Design review of the part shown in the three views and the two pictorial views. Dimensions are in mm from the part's minimum x, y and z. A direction names the side the tool comes from. Give positions to 0.01 mm unless a question says otherwise; leave off trailing zeros. Loops run counter-clockwise (first coordinate to the right, second up) from the corner with the lowest first, then second, coordinate; pieces in that order, holes last. Notation, with made-up numbers: (-22, 56.25) - (20, 56.25) arc R11 ccw to (20, 71.25) - close; hole circle Ø2 at (-36, 5). An arc over 180 degrees is marked (long way). Answer as a JSON object with one key per item and string values.
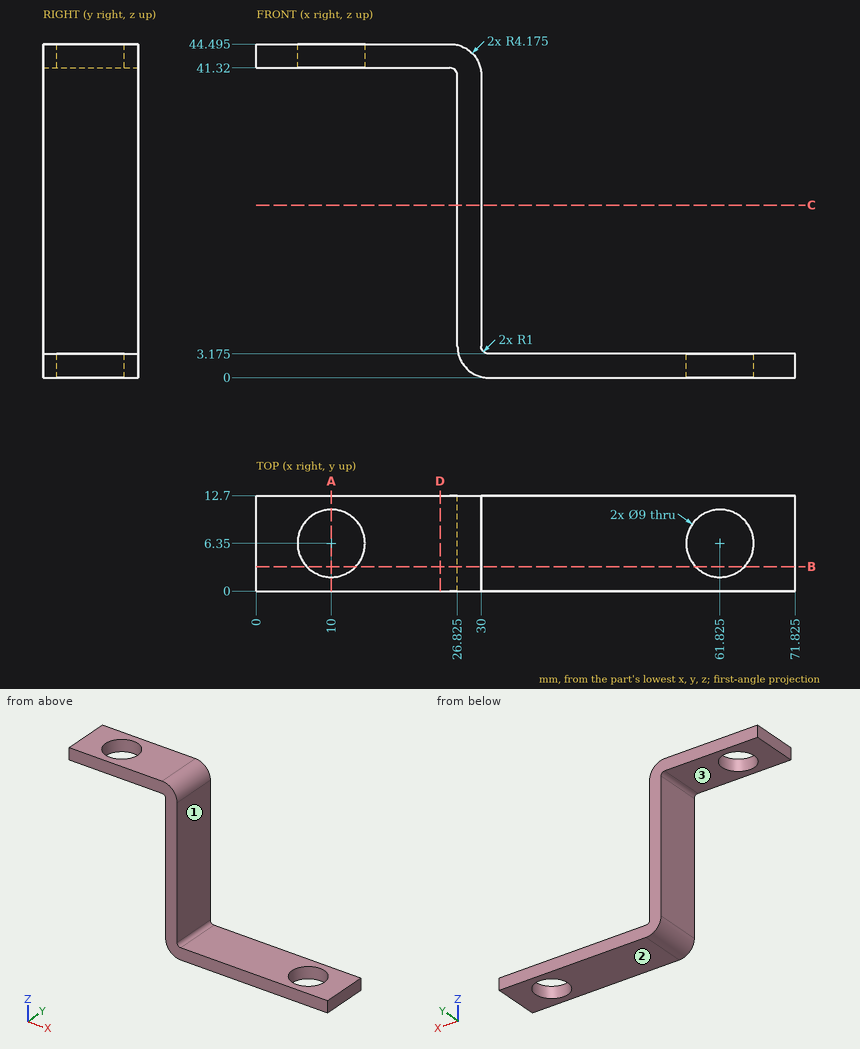
Q1. Consider section D-D, the plane x = 24.5. State the section outline as (y, z) points (3 decimals).
Results:
{"outline": "(0, 41.32) - (12.7, 41.32) - (12.7, 44.495) - (0, 44.495) - close"}
Q2. To check wall thickness, follow probe 1 along Y at (x, z) = (10, 42.2); probe 2 along X at (y, z) = (6, 32) (3 decimals); probe 3 along Z at (x, y) = (18.5, 2.75) (3 decimals). State the ranges of each line that lie inside material, in increasing order. Write a range as [from, to].
Results:
{"probe 1": "y = [0, 1.85], [10.85, 12.7]", "probe 2": "x = [26.825, 30]", "probe 3": "z = [41.32, 44.495]"}
Q3. Clearance check with flat-ended pins moving along their axes: pin 1 Ø6.5 at (y, z) = (6.5, 13.5) entering from -X (3 decimals); pin 2 Ø4 at (y, z) = (3.5, 17.5) entering from +X; pin 3 Ø5 at (x, y) = (22, 11.5) entering from -Z. State where each tip first meets the part, or that it passes through.
Results:
{"pin 1": "stops at x = 26.825", "pin 2": "stops at x = 30", "pin 3": "stops at z = 41.32"}
Q4. Consider section A-A, the plane x = 10. State the section outline as (y, z) points (3 decimals).
Results:
{"outline": "(0, 41.32) - (1.85, 41.32) - (1.85, 44.495) - (0, 44.495) - close; (10.85, 41.32) - (12.7, 41.32) - (12.7, 44.495) - (10.85, 44.495) - close"}
Q5. Consider section C-C, the plane z = 23. State the section outline as (x, y) points (3 decimals).
Results:
{"outline": "(26.825, 0) - (30, 0) - (30, 12.7) - (26.825, 12.7) - close"}
Q6. For the marked faces 1, 2 and 3, list the 3-axis set-ups (+Z, -Z, +X, -X, +Y, -Y) from which the entire face can be reached by the end or side of a thin tool; tool diameter is ignored.
Results:
{"face 1": "+Z, +X, +Y, -Y", "face 2": "-Z, +X, -X, +Y, -Y", "face 3": "-Z, -X, +Y, -Y"}
Q7. Consider section B-B, the plane y = 3.25. State the section outline as (x, z) points (3 decimals).
Results:
{"outline": "(0, 41.32) - (6.738, 41.32) - (6.738, 44.495) - (0, 44.495) - close; (13.262, 41.32) - (25.825, 41.32) arc R1 cw to (26.825, 40.32) - (26.825, 4.175) arc R4.175 ccw to (31, 0) - (58.563, 0) - (58.563, 3.175) - (31, 3.175) arc R1 cw to (30, 4.175) - (30, 40.32) arc R4.175 ccw to (25.825, 44.495) - (13.262, 44.495) - close; (65.087, 0) - (71.825, 0) - (71.825, 3.175) - (65.087, 3.175) - close"}
